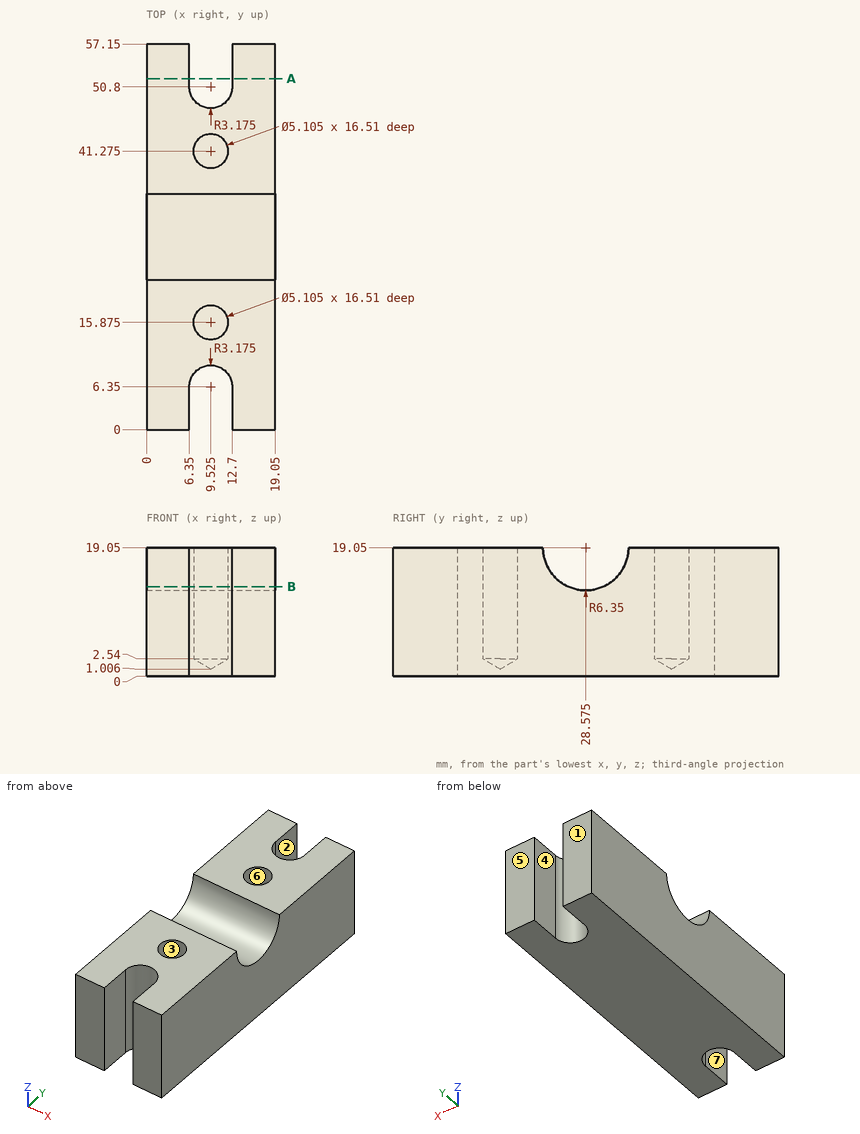
The figure shows three views and two pictorial views of one solid part (mm, origin at its lowest corner). Answer the questions. A direction names the side the tool comes from. Give positions to 0.01 mm unless a question says otherwise; leave off trailing zeros. Write each loop counter-clockwise with the first axis right and the second up, starting at its lowest first coordinate (ties: lowest second). Pieces come first, ordered by that corner, then holes. Notation, with made-up numbers: (4.25, -26) -> (14.25, -26) arc R27 ccw to (14.25, 1) -> close; hole circle Ø5 at (85, -34.75). An arc over 180 degrees is marked (long way). Use one line per item in the form item = value.
1) Each of these flat-tipped pins is pushed along its axis until it touches: P1, Ø3, axis at x = 9.525, y = 15.875, coming from the +Z side; P2, Ø4, axis at x = 4, z = 13, coming from the -Y side. Where does it stop, or does it pass through?
Result:
P1 = 1.91
P2 = 0
2) A tool of negligible diameter and unlimited length cuts with its end or side. For the marked faces 4, 5, 6 and 7, from which of +Z, -Z, +X, -X, +Y, -Y can it reach the whole face along a straight path? Write none if from no direction.
Result:
face_4 = +Z, -Z, +Y
face_5 = +Z, -Z, +X, -X, +Y
face_6 = +Z
face_7 = +Z, -Z, -Y
3) Section B-B on z = 13.25 is taken. Count the separate pieces of the cut face and the enclosed holes in it, plus the area to 3 significant figures.
Result:
separate_pieces = 2
enclosed_holes = 2
area = 837 mm²
4) For a pull along Y with two mould halves and no side action, classify the marked faces 1, 2 and 3 as +Y half, -Y half, draft (parallel to the pull), parting line (faces both ways), or undercut.
Result:
face_1 = +Y half
face_2 = draft
face_3 = undercut
5) Straight lines are drawn through the part: probe 1 along Y at (x, z) = (9.75, 11.5); probe 2 along Y at (x, z) = (8, 18.25) (1 decimal); probe 3 along X at (y, z) = (52, 10.25). For each, find the intervals that lie inside material, in ascending order.
Result:
probe_1 = 9.52 to 13.33, 18.42 to 38.73, 43.82 to 47.63
probe_2 = 9.1 to 13.8, 17.9 to 22.3, 34.9 to 39.2, 43.3 to 48
probe_3 = 0 to 6.35, 12.7 to 19.05
6) Section A-A on y = 52 is taken. Write down the section's boundary in (x, z), plus the area to 3 significant figures.
Result:
outline = (0, 0) -> (6.35, 0) -> (6.35, 19.05) -> (0, 19.05) -> close; (12.7, 0) -> (19.05, 0) -> (19.05, 19.05) -> (12.7, 19.05) -> close
area = 242 mm²
